Read the model definition and answer for the solid it produces. Units are mm, in the model's axes. Face numbers are marked on the shaded views. A direction names the side the tool comes from. Coordinates: 2 decimals unless noted, no trailing zeros. Write each loop counter-clockwise with the first axis right and the second up, starting at its lowest first coordinate (ties: lowest second). Pieces come first, ordered by that corner, then holes. Notation, with made-up numbers: (89, 29.25) -> (93, 29.25) arc R17 cw to (93, 58.25) -> close; hole circle Ø2 at (-28, 89.25). An arc over 180 degrees is marked (long way). Return JSON: item names as keys, results as strings.
from build123d import *

# Parameters (mm, degrees)
SKETCH_1_R          = 8.1
EXTRUDE_1_DEPTH     = 5
SKETCH_2_R          = 1.25
CUT_EXTRUDE_1_DEPTH = 5
SKETCH_3_R          = 1.25
CUT_EXTRUDE_2_DEPTH = 120
CHAMFER_1_SIZE      = 0.5
SKETCH_4_W          = 16
SKETCH_4_H          = 45
CUT_EXTRUDE_3_DEPTH = 10
FILLET_1_R          = 2
FILLET_2_R          = 15


with BuildPart() as part:
    # 草图1 → 凸台-拉伸1 (new body)
    with BuildSketch(Plane.XY):
        Polygon((4, 60), (4, 75), (0, 75), (0, 0), (4, 0), (4, 15), (70, 15), (70, 60), align=None)
        with Locations((20, 47)):
            Circle(SKETCH_1_R, mode=Mode.SUBTRACT)
    extrude(amount=EXTRUDE_1_DEPTH)

    # 草图2 → 切除-拉伸1 (cut)
    with BuildSketch(Plane(origin=(4, 0, 0), x_dir=(0, 0, -1), z_dir=(1, 0, 0))):
        with Locations((-2.5, 69)):
            Circle(SKETCH_2_R)
        with Locations((-2.5, 9)):
            Circle(SKETCH_2_R)
    extrude(amount=-CUT_EXTRUDE_1_DEPTH, mode=Mode.SUBTRACT)

    # 草图3 → 切除-拉伸2 (cut)
    with BuildSketch(Plane(origin=(0, 0, 0), x_dir=(-1, 0, 0), z_dir=(0, 0, -1))):
        with Locations((-40, 47)):
            Circle(SKETCH_3_R)
        with Locations((-20, 27)):
            Circle(SKETCH_3_R)
    extrude(amount=-CUT_EXTRUDE_2_DEPTH, mode=Mode.SUBTRACT)

    # 倒角1
    chamfer_1_edges = [part.edges().sort_by_distance(p)[0] for p in [
        (11.9, 47, 0),
        (11.9, 47, 5),
    ]]
    chamfer(chamfer_1_edges, length=CHAMFER_1_SIZE)

    # 草图4 → 切除-拉伸3 (cut)
    with BuildSketch(Plane(origin=(0, 0, 0), x_dir=(-1, 0, 0), z_dir=(0, 0, -1))):
        with Locations((-62, 37.5)):
            Rectangle(SKETCH_4_W, SKETCH_4_H)
    extrude(amount=-CUT_EXTRUDE_3_DEPTH, mode=Mode.SUBTRACT)

    # 圆角1
    fillet_1_edges = [part.edges().sort_by_distance(p)[0] for p in [
        (4, 75, 2.5),
        (4, 60, 2.5),
        (4, 15, 2.5),
        (4, 0, 2.5),
    ]]
    fillet(fillet_1_edges, radius=FILLET_1_R)

    # 圆角2
    fillet_2_edges = [part.edges().sort_by_distance(p)[0] for p in [
        (54, 60, 2.5),
        (54, 15, 2.5),
    ]]
    fillet(fillet_2_edges, radius=FILLET_2_R)


solid = part.part
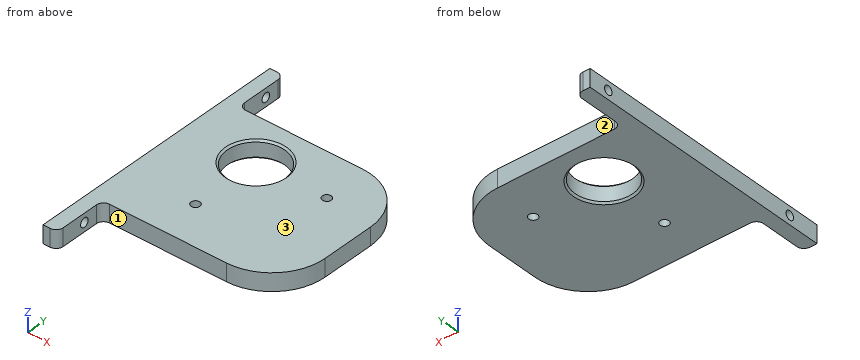
1. Flat-ended cylindrical pins translate along their axes: pin 1 Ø2 at (x, y) = (20, 27) entering from -Z; pin 2 Ø1.5 at (y, z) = (5, 2) entering from +X; pin 3 Ø2.5 at (x, z) = (30.5, 3.5) entering from -Y. Find the tip coordinate at first contact, or state that the pin passes through.
Taken from the geometry:
{"pin 1": "passes through", "pin 2": "stops at x = 4", "pin 3": "stops at y = 15"}
2. The part is cut by section B-B (x = 20). Determine the outline of the cut face in (y, z).
Taken from the geometry:
{"outline": "(15, 0) -> (25.75, 0) -> (25.75, 5) -> (15, 5) -> close; (28.25, 0) -> (38.4, 0) -> (38.9, 0.5) -> (38.9, 4.5) -> (38.4, 5) -> (28.25, 5) -> close; (55.1, 0.5) -> (55.6, 0) -> (60, 0) -> (60, 5) -> (55.6, 5) -> (55.1, 4.5) -> close"}
3. The part is cut by section C-C (x = 40). Determine the outline of the cut face in (y, z), then the cut area to 3 significant figures.
Taken from the geometry:
{"outline": "(15.03, 0) -> (45.75, 0) -> (45.75, 5) -> (15.03, 5) -> close; (48.25, 0) -> (59.97, 0) -> (59.97, 5) -> (48.25, 5) -> close", "area": "212 mm2"}
4. The part is cut by section A-A (y = 9). Determine the outline of the cut face in (x, z), then the cut area to 3 significant figures.
Taken from the geometry:
{"outline": "(0, 0) -> (4, 0) -> (4, 1.25) -> (0, 1.25) -> close; (0, 3.75) -> (4, 3.75) -> (4, 5) -> (0, 5) -> close", "area": "10.0 mm2"}
5. A tool of negligible diameter and unlimited length cuts with its end or side. For the marked faces 1, 2 and 3, from which of +Z, -Z, +X, -X, +Y, -Y can it reach the whole face along a straight path? Write none if from no direction.
Taken from the geometry:
{"face 1": "+Z, -Z, +X, -Y", "face 2": "+Z, -Z, +X, +Y", "face 3": "+Z, +X, -X, +Y, -Y"}
6. Consider L1, parallel to Y at x = 1.8, z = 2.5; L2, parallel to Y at x = 20, z = 1.5; L3, parallel to Z at x = 1.25, y = 69. Determine where each line is inside the solid, lowest interval first.
Taken from the geometry:
{"L1": "y = 0 to 7.75, 10.25 to 67.75, 70.25 to 75", "L2": "y = 15 to 25.75, 28.25 to 38.9, 55.1 to 60", "L3": "z = 0 to 1.25, 3.75 to 5"}
7. The part is cut by section D-D (y = 47). Determine the outline of the cut face in (x, z), then the cut area to 3 significant figures.
Taken from the geometry:
{"outline": "(0, 0) -> (11.4, 0) -> (11.9, 0.5) -> (11.9, 4.5) -> (11.4, 5) -> (0, 5) -> close; (28.1, 0.5) -> (28.6, 0) -> (38.75, 0) -> (38.75, 5) -> (28.6, 5) -> (28.1, 4.5) -> close; (41.25, 0) -> (53.87, 0) -> (53.87, 5) -> (41.25, 5) -> close", "area": "175 mm2"}
